Autodesk Inventor part; units mm, degrees
ref_plane "YZ Plane" through (0, 0, 0) normal (1, 0, 0) x (0, 1, 0)
ref_plane "XZ Plane" through (0, 0, 0) normal (0, 1, 0) x (-1, 0, 0)
ref_plane "XY Plane" through (0, 0, 0) normal (0, 0, 1) x (1, 0, 0)
sketch "Sketch1" plane through (0, 0, 0) normal (0, 1, 0) x (-1, 0, 0)
  circle A0 centre (0, 0) radius 4
  dimension "d0" = 8
extrude "Extrusion1" add sketch "Sketch1" along normal blind 360
sketch "Sketch2" plane through (0, 360, 0) normal (0, 1, 0) x (1, 0, 0)
  point P0 (0, 0)
hole "Hole1" at (0, 360, 0) direction (0, -1, 0) diameter 3.242 depth 20 tip angle 118
sketch "Sketch3" plane through (0, 0, 0) normal (0, -1, 0) x (1, 0, 0)
  point P0 (0, 0)
hole "Hole2" at (0, 0, 0) direction (0, 1, 0) diameter 3.242 depth 20 tip angle 118
properties part number "Stange_8mm_400mm"
Geometry check sheet. Reference: the model listing, model coordinates, mm. Give positions to 0.01 mm unless a question says otherwise; leave off trailing zeros. Loops run counter-clockwise (first coordinate to the right, second up) from the corner with the lowest first, then second, coordinate; pieces in that order, holes last. Notation, with made-up numbers: (60, -4.5) - (99, -4.5) arc R11 ccw to (99, -0.5) - close; hole circle Ø6 at (1, -8.75). An arc over 180 degrees is marked (long way). Use CSV: the item, a comma, the result in double quotes. Start each with the question number.
Q1. Section check A-A, the plane y = 249.5. Record the cut outline in (x, z), and give its area (3 significant figures).
Q2. Scan lines: probe 1 along Z at (x, y) = (0, 14.5); probe 2 along Z at (x, y) = (0.75, 183); probe 3 along X at (y, z) = (60, 0.25). Record each from-to range of solid material in increasing order. Write a range as from..to.
Q3. Go/stop test with a flat-tipped pin: pin 1 Ø2 at (x, y) = (2.5, 130.5) entering from -Z. Record where the tip stops, or that it passes through.
Findings below:
1,outline,"circle Ø8 at (0, 0)"
1,area,"50.3 mm^2"
2,probe 1,"z = -4..-1.62, 1.62..4"
2,probe 2,"z = -3.93..3.93"
2,probe 3,"x = -3.99..3.99"
3,pin 1,"stops at z = -3.71"
